Part model, mm, in its own coordinate system. A direction names the side the tool comes from. Coordinates: 2 decimals unless noted, no trailing zeros. Loops run counter-clockwise (first coordinate to the right, second up) from the corner with the lowest first, then second, coordinate; pieces in that order, holes last.
```python
from build123d import *

# Parameters (mm, degrees)
SKETCH1_R           = 12.5
SKETCH1_R_2         = 4
BOSS_EXTRUDE1_DEPTH = 2.5
SKETCH2_W           = 25
SKETCH2_H           = 5
SKETCH2_W_2         = 5
BOSS_EXTRUDE3_DEPTH = 40
SKETCH3_W           = 35
SKETCH3_H           = 10
BOSS_EXTRUDE5_DEPTH = 29.5
SKETCH5_R           = 12.25
CUT_EXTRUDE1_DEPTH  = 29.5
SKETCH6_R           = 1.5
CUT_EXTRUDE2_DEPTH  = 29.5
SKETCH7_R           = 1.475
CUT_EXTRUDE4_DEPTH  = 10
SKETCH8_R           = 1.5
CUT_EXTRUDE5_DEPTH  = 10


with BuildPart() as part:
    # Sketch1 → Boss-Extrude1 (new body)
    with BuildSketch(Plane.XY):
        with BuildLine():
            Line((12.5, 20), (-12.5, 20))
            Line((-12.5, 20), (-12.5, 1.2e-08))
            ThreePointArc((-12.5, 1.2e-08), (6e-09, 12.5), (12.5, 0))
            Line((12.5, 0), (12.5, 20))
        make_face()
        Circle(SKETCH1_R)
        Circle(SKETCH1_R_2, mode=Mode.SUBTRACT)
    extrude(amount=BOSS_EXTRUDE1_DEPTH)

    # Sketch2 → Boss-Extrude3 (add)
    with BuildSketch(Plane(origin=(0, 0, 0), x_dir=(-1, 0, 0), z_dir=(0, 0, -1))):
        with Locations((0, 17.5)):
            Rectangle(SKETCH2_W, SKETCH2_H)
        with Locations((-15, 17.5)):
            Rectangle(SKETCH2_W_2, SKETCH2_H)
        with Locations((15, 17.5)):
            Rectangle(SKETCH2_W_2, SKETCH2_H)
    extrude(amount=-BOSS_EXTRUDE3_DEPTH)

    # Sketch3 → Boss-Extrude5 (add)
    with BuildSketch(Plane.XZ.offset(-15)):
        with Locations((0, 35)):
            Rectangle(SKETCH3_W, SKETCH3_H)
    extrude(amount=BOSS_EXTRUDE5_DEPTH)

    # Sketch5 → Cut-Extrude1 (cut)
    with BuildSketch(Plane(origin=(0, 0, 30), x_dir=(-1, 0, 0), z_dir=(0, 0, -1))):
        Circle(SKETCH5_R)
        with BuildLine():
            Line((17.5, -14.5), (17.5, -4.5))
            ThreePointArc((17.5, -4.5), (14.571067812, -11.571067812), (7.5, -14.5))
            Line((7.5, -14.5), (17.5, -14.5))
        make_face()
        with BuildLine():
            ThreePointArc((-7.5, -14.5), (-14.571067812, -11.571067812), (-17.5, -4.5))
            Line((-17.5, -4.5), (-17.5, -14.5))
            Line((-17.5, -14.5), (-7.5, -14.5))
        make_face()
    extrude(amount=-CUT_EXTRUDE1_DEPTH, mode=Mode.SUBTRACT)

    # Sketch6 → Cut-Extrude2 (cut)
    with BuildSketch(Plane(origin=(0, 0, 0), x_dir=(-1, 0, 0), z_dir=(0, 0, -1))):
        with Locations((0, 8.5)):
            Circle(SKETCH6_R)
        with Locations((0, -8.5)):
            Circle(SKETCH6_R)
    extrude(amount=-CUT_EXTRUDE2_DEPTH, mode=Mode.SUBTRACT)

    # Sketch7 → Cut-Extrude4 (cut)
    with BuildSketch(Plane.XZ.offset(-15)):
        with Locations((7.5, 23)):
            Circle(SKETCH7_R)
        with Locations((-7.5, 23)):
            Circle(SKETCH7_R)
        with Locations((7.5, 9.5)):
            Circle(SKETCH7_R)
        with Locations((-7.5, 9.5)):
            Circle(SKETCH7_R)
    extrude(amount=-CUT_EXTRUDE4_DEPTH, mode=Mode.SUBTRACT)

    # Sketch8 → Cut-Extrude5 (cut)
    with BuildSketch(Plane(origin=(0, 0, 0), x_dir=(-1, 0, 0), z_dir=(0, 0, -1))):
        with Locations((-8.5, 0)):
            Circle(SKETCH8_R)
        with Locations((8.5, 0)):
            Circle(SKETCH8_R)
    extrude(amount=-CUT_EXTRUDE5_DEPTH, mode=Mode.SUBTRACT)


solid = part.part
```
Q1. Saw through at D-D (y = 18). List the corners of the cut face in (x, z) (3 decimals), plus the area to 3 significant figures.
Q2. Saw through at B-B (x = 0). List the corners of the cut face in (y, z), plus the area to 3 significant figures.
Q3. Tool access for faces 4 (the flat face through (12.5, 7, 1)), 5 (the cylindrical face through (-6.586, 10.329, 34.93)), 6 (the flat face through (-12, 4, 30)): list every direction of +Z, -Z, +X, -X, +Y, -Y with a clear straight run to the whole face (end or side of a thin tool).
Q4. Saw through at C-C (z = 9.5). List the corners of the cut face in (x, y) (3 decimals), plus the area to 4 significant figures.
Q5. Saw through at A-A (y = 6). List the corners of the cut face in (x, z).
Q6. Drop flat-ended pins along their axis: P1, Ø8, axis at x = 1, y = 0.5, coming from the +Z side; P2, Ø2, axis at y = 6.5, z = 1.5, coming from the -X side; P3, Ø1.8, axis at x = 8.5, y = 0, coming from the -Z side; P4, Ø3.5, axis at x = -7.5, z = 23, coming from the -Y side. Give the stop position or say it passes through.
Q7. Mould opens along Z. For faces 1 (the flat face through (0, 14, 40)), 2 (the cylindrical face through (7.18, 17.46, 21.56)), 3 (the cylindrical face through (0, -10, 1)) say: released by +Z, released by -Z, zero draft, split by the parting line, or undercut.
Q8. Probe line 1 (Z direction, x = 7.5, y = 16.05) (3 decimals); line 2 (Y direction, x = 0, z = 1); line 3 (Y direction, x = 12.5, z = 6.5). List the from-to ranges inside material, lowest first.
Checked values:
1. outline: (-17.5, 0) - (17.5, 0) - (17.5, 40) - (-17.5, 40) - close; hole circle Ø2.95 at (-7.5, 9.5); hole circle Ø2.95 at (-7.5, 23); hole circle Ø2.95 at (7.5, 9.5); hole circle Ø2.95 at (7.5, 23)
1. area: 1,370 mm2
2. outline: (-14.5, 30) - (-12.25, 30) - (-12.25, 40) - (-14.5, 40) - close; (-12.5, 0) - (-10, 0) - (-10, 2.5) - (-12.5, 2.5) - close; (-7, 0) - (-4, 0) - (-4, 2.5) - (-7, 2.5) - close; (4, 0) - (7, 0) - (7, 2.5) - (4, 2.5) - close; (10, 0) - (20, 0) - (20, 40) - (12.25, 40) - (12.25, 30) - (15, 30) - (15, 2.5) - (10, 2.5) - close
2. area: 284 mm2
3. face 4: -Z, +X, -Y
3. face 5: +Z
3. face 6: +X, -X, -Y
4. outline: (-17.5, 15) - (-8.975, 15) - (-8.975, 20) - (-17.5, 20) - close; (-6.025, 15) - (6.025, 15) - (6.025, 20) - (-6.025, 20) - close; (8.975, 15) - (17.5, 15) - (17.5, 20) - (8.975, 20) - close
4. area: 145.5 mm2
5. outline: (-17.5, 30) - (-10.68, 30) - (-10.68, 40) - (-17.5, 40) - close; (-12.5, 0) - (12.5, 0) - (12.5, 2.5) - (-12.5, 2.5) - close; (10.68, 30) - (17.5, 30) - (17.5, 40) - (10.68, 40) - close
6. P1: stops at z = 2.5
6. P2: stops at x = -12.5
6. P3: passes through
6. P4: stops at y = 15
7. face 1: released by +Z
7. face 2: undercut
7. face 3: zero draft
8. line 1: z = 0 to 8.025, 10.975 to 21.525, 24.475 to 40
8. line 2: y = -12.5 to -10, -7 to -4, 4 to 7, 10 to 20
8. line 3: y = 15 to 20
